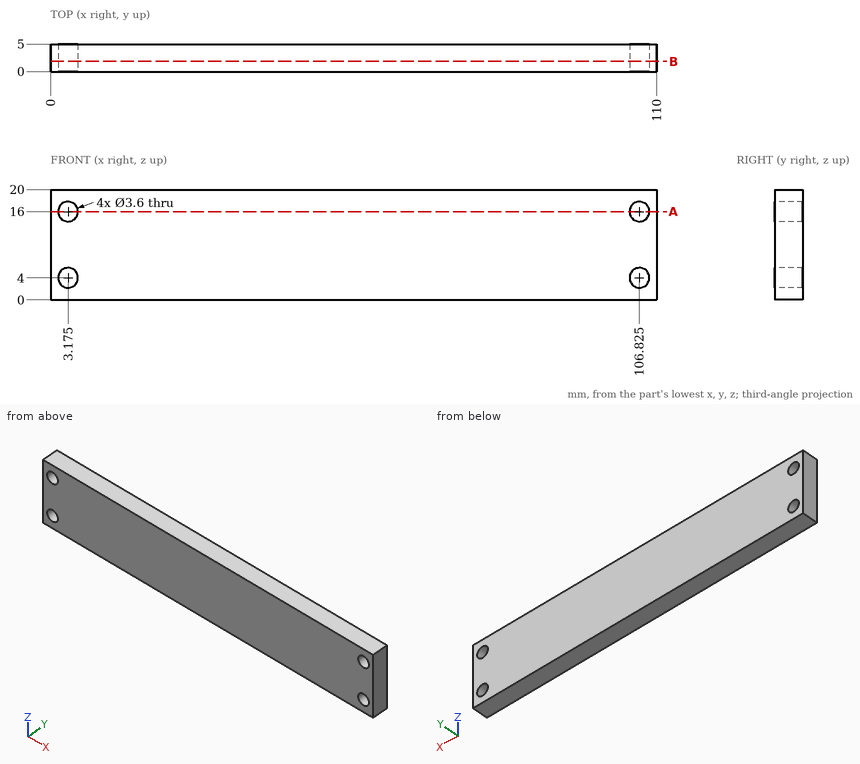
The drawing under review shows one solid part. Ordinate dimensions are in mm from its lowest x, y, z. Give positions to 0.01 mm unless a question says otherwise; leave off trailing zeros. Loops run counter-clockwise (first coordinate to the right, second up) from the corner with the lowest first, then second, coordinate; pieces in that order, holes last. Notation, with made-up numbers: M -1,27.25 L 24,27.25 A32 cw 24,61.25 Z; hole C -31.5,49.5 d6. An arc over 180 degrees is marked long. One line per question, with ' | ' between items. Start each with the question number.
1. Insertion check: P1, Ø3, axis at x = 3.175, z = 4, coming from the -Y side. The pin has a flat end and moves straight along its axis. Give the tip position at first contact, or say it passes through.
2. Add section A-A (z = 16). Write out the cut boundary in (x, y) (3 decimals).
3. Add section B-B (y = 1.85). Write out the cut boundary in (x, z) (3 decimals), plus the area to 3 significant figures.
4. To check wall thickness, follow L1, parallel to X at y = 2.05, z = 16 (3 decimals); L2, parallel to X at y = 1.9, z = 5.25. State the ranges of each line that lie inside material, in increasing order.
Worked out:
1) P1: passes through
2) outline: M 0,0 L 1.375,0 L 1.375,5 L 0,5 Z; M 4.975,0 L 105.025,0 L 105.025,5 L 4.975,5 Z; M 108.625,0 L 110,0 L 110,5 L 108.625,5 Z
3) outline: M 0,0 L 110,0 L 110,20 L 0,20 Z; hole C 3.175,4 d3.6; hole C 3.175,16 d3.6; hole C 106.825,4 d3.6; hole C 106.825,16 d3.6 | area: 2,160 mm²
4) L1: x = 0 to 1.375, 4.975 to 105.025, 108.625 to 110 | L2: x = 0 to 1.88, 4.47 to 105.53, 108.12 to 110
